Work out the finished part from the listing and answer in its coordinate system (mm). Face numbers are marked on the shaded views. Coordinates: 2 decimals unless noted, no trailing zeros. Order: outer loops, then holes, each group sorted by start corner. A loop starts at its lowest first (then second) coordinate and runs counter-clockwise, first axis right, second up. Notation, with made-up numbers: (1, 0.5) - (47, 0.5) arc R20 cw to (47, 36.5) - close; hole circle Ø10 at (-25.75, -1). An arc over 180 degrees is marked (long way). Use CSV: the item, a comma, the result in double quotes. Start each with the question number.
from build123d import *

# Parameters (mm, degrees)
BOSS_EXTRUDE1_DEPTH = 2.38125
SKETCH2_R           = 7.5
CUT_EXTRUDE1_DEPTH  = 0.1


with BuildPart() as part:
    # Sketch1 → Boss-Extrude1 (new body)
    with BuildSketch(Plane(origin=(0, 0, 0), x_dir=(1, 0, 0), z_dir=(0, 1, 0))):
        with BuildLine():
            Line((-8.357145147, 31.238774815), (-31.232145147, -8.381887408))
            ThreePointArc((-31.232145147, -8.381887408), (-31.232145147, -18.031887408), (-22.875, -22.856887408))
            Line((-22.875, -22.856887408), (22.875, -22.856887408))
            ThreePointArc((22.875, -22.856887408), (31.232145147, -18.031887408), (31.232145147, -8.381887408))
            Line((31.232145147, -8.381887408), (8.357145147, 31.238774815))
            ThreePointArc((8.357145147, 31.238774815), (0, 36.063774815), (-8.357145147, 31.238774815))
        make_face()
    extrude(amount=BOSS_EXTRUDE1_DEPTH)

    # Sketch2 → Cut-Extrude1 (cut)
    with BuildSketch(Plane(origin=(0, 2.38125, 0), x_dir=(1, 0, 0), z_dir=(0, 1, 0))):
        with Locations((0, 9.613774815)):
            Circle(SKETCH2_R)
    extrude(amount=-CUT_EXTRUDE1_DEPTH, mode=Mode.SUBTRACT)


solid = part.part
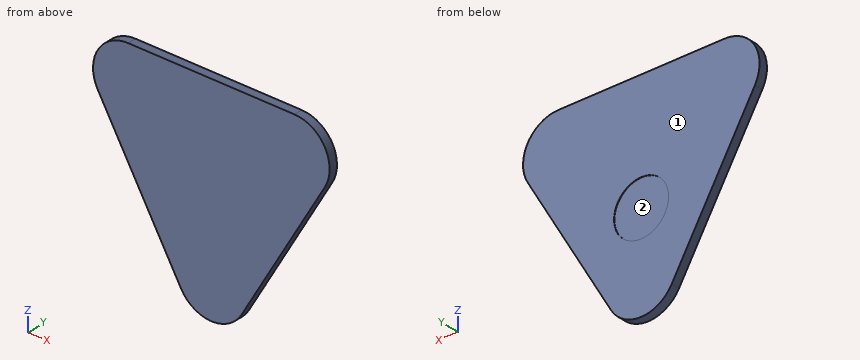
1) The part is cut by section B-B on z = -13. Determine the outline of the cut face in (x, y).
2) The part is cut by section C-C on x = -25.5. Determine the outline of the cut face in (y, z).
3) The part is cut by section D-D on x = 28. Determine the outline of the cut face in (y, z).
4) Straight lines are drawn through the part: line 1 (Y direction, x = -4, z = -7); line 2 (X direction, y = 0.85, z = 15.5); line 3 (Z direction, x = -27, y = 1.3). For each, find the intervals that lie inside material, in ascending order. Write a range as [from, to].
5) The part is cut by section A-A on y = 1.05. Determine the outline of the cut face in (x, z) (3 decimals).
6) For a pull along Z with two mould halves and no side action, classify the marked faces 1 and 2 as +Z half, -Z half, draft (parallel to the pull), parting line (faces both ways), or undercut.
Answer key:
1,outline,"(-18.89, 0) - (18.89, 0) - (18.89, 2.38) - (6.69, 2.38) - (6.69, 2.28) - (-6.69, 2.28) - (-6.69, 2.38) - (-18.89, 2.38) - close"
2,outline,"(0, -1.55) - (2.38, -1.55) - (2.38, 22.49) - (0, 22.49) - close"
3,outline,"(0, 2.78) - (2.38, 2.78) - (2.38, 21.38) - (0, 21.38) - close"
4,line 1,"[0, 2.28]"
4,line 2,"[-32.25, 32.25]"
4,line 3,"[1.05, 21.93]"
5,outline,"(-31.232, 8.382) - (-8.357, -31.239) arc R9.65 ccw to (8.357, -31.239) - (31.232, 8.382) arc R9.65 ccw to (22.875, 22.857) - (-22.875, 22.857) arc R9.65 ccw to start"
6,face 1,"draft"
6,face 2,"undercut"
